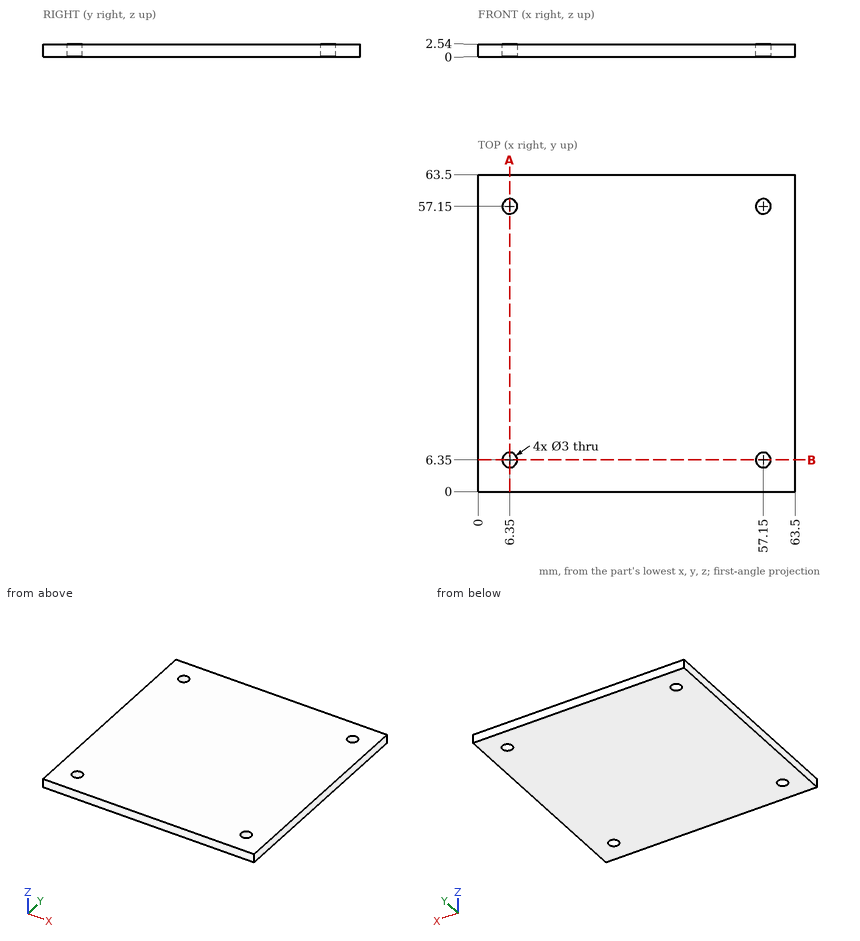
For this review, use the dimensioned drawing (mm, ordinates from the lowest corner) and the shaded views. Coordinates: 2 decimals unless noted, no trailing zeros. Loops run counter-clockwise (first coordinate to the right, second up) from the corner with the lowest first, then second, coordinate; pieces in that order, holes last. Notation, with made-up numbers: (44, 39.5) -> (86, 39.5) arc R13 ccw to (86, 64.5) -> close; hole circle Ø3 at (-24, 87). An arc over 180 degrees is marked (long way). Use a Markdown table: item, result. Add a question column.
Item 1: Clearance check with flat-ended pins moving along their axes: P1, Ø6, axis at x = 12.5, y = 44, coming from the -Z side; P2, Ø2.5, axis at x = 57.15, y = 6.35, coming from the -Z side. State where each tip first meets the part, or that it passes through.
Item 2: We need section A-A, the plane x = 6.35. Write out the cut boundary in (y, z), and give its area (3 significant figures).
Item 3: Wall thickness on L1, parallel to Y at x = 6.35, z = 0.7; L2, parallel to Y at x = 58, z = 1.6: over which ranges is each line inside the solid? List them lowest first. Write a range as from..to.
Numbers:
| question | item | result |
|---|---|---|
| 1 | P1 | stops at z = 0 |
| 1 | P2 | passes through |
| 2 | outline | (0, 0) -> (4.85, 0) -> (4.85, 2.54) -> (0, 2.54) -> close; (7.85, 0) -> (55.65, 0) -> (55.65, 2.54) -> (7.85, 2.54) -> close; (58.65, 0) -> (63.5, 0) -> (63.5, 2.54) -> (58.65, 2.54) -> close |
| 2 | area | 146 mm^2 |
| 3 | L1 | y = 0..4.85, 7.85..55.65, 58.65..63.5 |
| 3 | L2 | y = 0..5.11, 7.59..55.91, 58.39..63.5 |
